from build123d import *

# Parameters (mm, degrees)
F0_R     = 2.667
F1_DEPTH = 3.175
F2_DEPTH = 48.641


with BuildPart() as f1:
    # F0 (on Front) → F1 (new body)
    with BuildSketch(Plane.XZ):
        Polygon((2.566322, 4.445), (-2.566322, 4.445), (-5.132644, 0), (-2.566322, -4.445), (2.566322, -4.445), (5.132644, 0), align=None)
        Circle(F0_R, mode=Mode.SUBTRACT)
        Circle(F0_R)
    extrude(amount=F1_DEPTH)

    # F0 (on Front) → F2 (join)
    with BuildSketch(Plane.XZ):
        Circle(F0_R)
    extrude(amount=F2_DEPTH)


solid = f1.part
Design review of the part built by this model. Coordinates are the model's own, in mm. A direction names the side the tool comes from. Coordinates: 2 decimals unless noted, no trailing zeros. Write each loop counter-clockwise with the first axis right and the second up, starting at its lowest first coordinate (ties: lowest second). Pieces come first, ordered by that corner, then holes. Notation, with made-up numbers: (27.5, -23.75) - (34.5, -23.75) arc R19 cw to (34.5, -8.75) - close; hole circle Ø6 at (0, 12.5). An arc over 180 degrees is marked (long way). Use one line per item in the form item = value.
Q1. Consider section C-C (z = 2.25). Write out the cut boundary in (x, y) (3 decimals).
Taken from the geometry:
outline = (-3.834, -3.175) - (-1.432, -3.175) - (-1.432, -48.641) - (1.432, -48.641) - (1.432, -3.175) - (3.834, -3.175) - (3.834, 0) - (-3.834, 0) - close
Q2. Consider section D-D (z = -3.25). Write out the cut boundary in (x, y) (3 decimals), plus the area to 3 significant figures.
Taken from the geometry:
outline = (-3.256, -3.175) - (3.256, -3.175) - (3.256, 0) - (-3.256, 0) - close
area = 20.7 mm^2
Q3. Insertion check: pin 1 Ø1 at (y, z) = (-13, 0.5) entering from +X; pin 2 Ø1.5 at (x, y) = (0, -29) entering from -Z; pin 3 Ø1.5 at (y, z) = (-27.5, 2.5) entering from -X; pin 4 Ø1.5 at (x, y) = (4, -43) entering from -Z. Each pin has a flat end and moves straight along its axis. Give the tip position at first contact, or say it passes through.
Taken from the geometry:
pin_1 = 2.67
pin_2 = -2.67
pin_3 = -2.01
pin_4 = through
Q4. Consider section B-B (y = -35.5). Write out the cut boundary in (x, z).
Taken from the geometry:
outline = circle Ø5.33 at (0, 0)
Q5. Machinability: for faces 1 (the flat face through (-3.87, -1.57, -2.19)), 2 (the cylindrical face through (1.231, -25.59, -2.366)), which of the approach directions +Z, -Z, +X, -X, +Y, -Y give a long, thin tool a straight path to every point of the face, cutting with its end or side? Answer none if there is none.
Taken from the geometry:
face_1 = -Z, -X, +Y, -Y
face_2 = -Y
Q6. Consider section A-A (x = 0). Write out the cut boundary in (y, z) (3 decimals), plus the area to 3 significant figures.
Taken from the geometry:
outline = (-48.641, -2.667) - (-3.175, -2.667) - (-3.175, -4.445) - (0, -4.445) - (0, 4.445) - (-3.175, 4.445) - (-3.175, 2.667) - (-48.641, 2.667) - close
area = 271 mm^2
Q7. For probe 1 along Y at (x, z) = (3, 3.25) (3 decimals); probe 2 along X at (y, z) = (-24.5, 0.75), list the stretches that pass through material, from the lowest coordinate up.
Taken from the geometry:
probe_1 = -3.175 to 0
probe_2 = -2.56 to 2.56
